from build123d import *

# Parameters (mm, degrees)
ESQUISSE1_W             = 50
ESQUISSE1_H             = 50
BOSS_EXTRU_1_DEPTH      = 50
ESQUISSE2_R             = 6
ENL_V_MAT_EXTRU_1_DEPTH = 40
CONG_1_R                = 10
ESQUISSE3_R             = 1.5
ENL_V_MAT_EXTRU_2_DEPTH = 15
ENL_V_MAT_EXTRU_3_DEPTH = 5


with BuildPart() as part:
    # Esquisse1 → Boss.-Extru.1 (new body)
    with BuildSketch(Plane.XY):
        with Locations((25, 25)):
            Rectangle(ESQUISSE1_W, ESQUISSE1_H)
    extrude(amount=BOSS_EXTRU_1_DEPTH)

    # Esquisse2 → Enlèv. mat.-Extru.1 (cut)
    with BuildSketch(Plane.ZY):
        with Locations((24.976890997, 24.856256207)):
            Circle(ESQUISSE2_R)
    extrude(amount=-ENL_V_MAT_EXTRU_1_DEPTH, mode=Mode.SUBTRACT)

    # Congé1
    cong_1_edges = [part.edges().sort_by_distance(p)[0] for p in [
        (25, 50, 50),
        (25, 50, 0),
        (25, 0, 0),
        (25, 0, 50),
    ]]
    fillet(cong_1_edges, radius=CONG_1_R)

    # Esquisse3 → Enlèv. mat.-Extru.2 (cut)
    with BuildSketch(Plane(origin=(0, 50, 0), x_dir=(1, 0, 0), z_dir=(0, 1, 0))):
        with Locations(Location((10.546738136, -14.940962314, 0), (0, 0, 270))):
            Circle(ESQUISSE3_R)
    extrude(amount=-ENL_V_MAT_EXTRU_2_DEPTH, mode=Mode.SUBTRACT)

    # Esquisse4 → Enlèv. mat.-Extru.3 (cut)
    with BuildSketch(Plane(origin=(50, 0, 0), x_dir=(0, 0, -1), z_dir=(1, 0, 0))):
        with BuildLine():
            Line((-19.291182269, 32.286465455), (-21.302414692, 42.065190949))
            ThreePointArc((-21.302414692, 42.065190949), (-24.926554612, 45.019798544), (-28.550694532, 42.065190949))
            Line((-28.550694532, 42.065190949), (-30.561926955, 32.286465455))
            ThreePointArc((-30.561926955, 32.286465455), (-31.290515643, 30.383759574), (-33.193221523, 29.655170887))
            Line((-33.193221523, 29.655170887), (-42.971947017, 27.643938464))
            ThreePointArc((-42.971947017, 27.643938464), (-45.926554612, 24.019798544), (-42.971947017, 20.395658623))
            Line((-42.971947017, 20.395658623), (-33.193221523, 18.384426201))
            ThreePointArc((-33.193221523, 18.384426201), (-31.290515643, 17.655837513), (-30.561926955, 15.753131632))
            Line((-30.561926955, 15.753131632), (-28.550694532, 5.974406139))
            ThreePointArc((-28.550694532, 5.974406139), (-28.155011664, 4.912296106), (-27.45637674, 4.019798544))
            ThreePointArc((-27.45637674, 4.019798544), (-24.926554612, 3.123395403), (-22.396732484, 4.019798544))
            ThreePointArc((-22.396732484, 4.019798544), (-21.69809756, 4.912296106), (-21.302414692, 5.974406139))
            Line((-21.302414692, 5.974406139), (-19.291182269, 15.753131632))
            ThreePointArc((-19.291182269, 15.753131632), (-18.562593581, 17.655837513), (-16.6598877, 18.384426201))
            Line((-16.6598877, 18.384426201), (-6.881162207, 20.395658623))
            ThreePointArc((-6.881162207, 20.395658623), (-3.926554612, 24.019798544), (-6.881162207, 27.643938464))
            Line((-6.881162207, 27.643938464), (-16.6598877, 29.655170887))
            ThreePointArc((-16.6598877, 29.655170887), (-18.562593581, 30.383759574), (-19.291182269, 32.286465455))
        make_face()
    extrude(amount=-ENL_V_MAT_EXTRU_3_DEPTH, mode=Mode.SUBTRACT)


solid = part.part
Could you check a few things on this model? Use its own coordinates, in mm. A direction names the side the tool comes from. Give positions to 0.01 mm unless a question says otherwise; leave off trailing zeros. Order: outer loops, then holes, each group sorted by start corner. A loop starts at its lowest first (then second) coordinate and runs counter-clockwise, first axis right, second up. Notation, with made-up numbers: (-15, 65) -> (20, 65) arc R13 cw to (20, 70) -> close; hole circle Ø11 at (50.5, -8). An arc over 180 degrees is marked (long way). Answer in a Markdown table with one row per item. Add a question column.
Item 1: Please list where these lines run through material, in increasing order: probe 1 along Y at (x, z) = (24.5, 25); probe 2 along X at (y, z) = (27, 11.5); probe 3 along X at (y, z) = (30.5, 24).
Item 2: Imagine slicing it at A-A (x = 41). List the corners of the cut face in (y, z) for me, and give its area (3 significant figures).
Item 3: Imagine slicing it at B-B (z = 15.5). List the corners of the cut face in (x, y) for me.
Item 4: For faces 4 (the flat face through (25, 50, 25)), 5 (the cylindrical face through (47.535, 17.676, 31.311)), 6 (the flat face through (40, 25, 25)), which set-ups out of +Z, -Z, +X, -X, +Y, -Y let a thin tool reach every point of the face, with its end or its side?
Item 5: I'm going to push flat-ended pins straight in: P1, Ø9.5, axis at y = 24.86, z = 24.98, coming from the +X side; P2, Ø1.5, axis at x = 10.5, z = 15, coming from the +Y side; P3, Ø1, axis at x = 6, z = 43.5, coming from the +Y side. Where does each tip first touch, or does it pass through?
Item 6: Imagine slicing it at D-D (x = 31.5). List the corners of the cut face in (y, z) for me, and give its area (3 significant figures).
Item 7: We'd pull the mould along Z, two halves only. Please class faces 1 (the flat face through (47.535, 19.404, 38.151)), 2 (the flat face through (25, 25, 0)), 3 (the flat face through (25, 0, 25)): pulls with the +Z half, pulls with the -Z half, needs draft (parallel to the pull), parting line crosses it, or undercut.
Item 8: Imagine slicing it at C-C (y = 16.5). List the corners of the cut face in (x, z) for me.
Result:
| question | item | result |
|---|---|---|
| 1 | probe 1 | 0 to 18.86, 30.86 to 50 |
| 1 | probe 2 | 0 to 45 |
| 1 | probe 3 | 40 to 45 |
| 2 | outline | (0, 10) arc R10 ccw to (10, 0) -> (40, 0) arc R10 ccw to (50, 10) -> (50, 40) arc R10 ccw to (40, 50) -> (10, 50) arc R10 ccw to (0, 40) -> close |
| 2 | area | 2,410 mm2 |
| 3 | outline | (0, 0) -> (50, 0) -> (50, 18.62) -> (45, 18.62) -> (45, 29.42) -> (50, 29.42) -> (50, 50) -> (11.94, 50) -> (11.94, 35) -> (9.15, 35) -> (9.15, 50) -> (0, 50) -> close |
| 4 | face 4 | +Z, -Z, +X, -X, +Y |
| 4 | face 5 | +X |
| 4 | face 6 | -X |
| 5 | P1 | x = 45 |
| 5 | P2 | y = 35 |
| 5 | P3 | y = 49.54 |
| 6 | outline | (0, 10) arc R10 ccw to (10, 0) -> (40, 0) arc R10 ccw to (50, 10) -> (50, 40) arc R10 ccw to (40, 50) -> (10, 50) arc R10 ccw to (0, 40) -> close; hole circle Ø12 at (24.86, 24.98) |
| 6 | area | 2,300 mm2 |
| 7 | face 1 | undercut |
| 7 | face 2 | pulls with the -Z half |
| 7 | face 3 | needs draft |
| 8 | outline | (0, 0) -> (50, 0) -> (50, 19.22) -> (45, 19.22) -> (45, 30.63) -> (50, 30.63) -> (50, 50) -> (0, 50) -> close |
